Here's how the part is built. I have some questions about the finished solid (model axes, mm). A direction names the side the tool comes from. Coordinates: 2 decimals unless noted, no trailing zeros. Write each loop counter-clockwise with the first axis right and the second up, starting at its lowest first coordinate (ties: lowest second). Pieces come first, ordered by that corner, then holes. Notation, with made-up numbers: (-38, 89.5) -> (-13, 89.5) arc R16 cw to (-13, 115.5) -> close; hole circle Ø6 at (-14.75, 13.5). An arc over 180 degrees is marked (long way). Use a Markdown table: item, result. Add a question column.
Item 1: Will these pins go through, and if not, where does the flat tip stop? pin 1 Ø1.6 at (x, y) = (73.5, 70) entering from +Z; pin 2 Ø3.5 at (x, y) = (14.5, 61.2) entering from +Z.
Item 2: Imagine slicing it at D-D, the plane x = 60.5. Write out the boundary of the cut face in (y, z).
Item 3: Imagine slicing it at A-A, the plane y = -3. Write out the boundary of the cut face in (x, z), and give its area (3 significant figures).
Item 4: If I drill on line 1 along Y through (x, z) = (14.5, 2.6) (3 decimals); line 2 along X through (y, z) = (35.65, 3.3); line 3 along X through (y, z) = (52, 1.85), over which ranges is the centre line in solid material (lowest first)? Write a range as from..to.
Item 5: On a 3-axis mill with a long thin cutter (end or side, diameter ignored), from which of +Z, -Z, +X, -X, +Y, -Y can I reach the whole of each face in a straight line? I mean faces 1 (the flat face through (45, -6, 5.4)), 2 (the cylindrical face through (9.34, 7.52, 2.94)), 3 (the cylindrical face through (85.9, 9.93, 2.74)). Say none if no direction works.
Item 6: Imagine slicing it at C-C, the plane y = 21.65. Write out the boundary of the cut face in (x, z).
Item 7: If we mould it in two halves opening along X, with no side actions, what happens to faces 4 (the flat face through (64, 10.5, 3)), 5 (the flat face through (60, 47, 5.4))? For each: pulls with the +X half, pulls with the -X half, needs draft (parallel to the pull), parting line crosses it, or undercut.
Item 8: Imagine slicing it at B-B, the plane z = 2.4. Count the separate pieces of the cut face and the enclosed holes in it, and give its area (3 significant figures).
```python
from build123d import *

# Parameters (mm, degrees)
SKETCH1_R           = 2.75
SKETCH1_R_2         = 2.25
BOSS_EXTRUDE1_DEPTH = 5.4
FILLET1_R           = 4
SKETCH2_R           = 3.025
CUT_EXTRUDE1_DEPTH  = 6.4
SKETCH3_R           = 2.25
CUT_EXTRUDE2_DEPTH  = 5
CIRPATTERN1_COUNT   = 2
FILLET2_R           = 2
FILLET3_R           = 2
SKETCH5_W           = 99
SKETCH5_H           = 83.2
SKETCH5_W_2         = 93
SKETCH5_H_2         = 77.2
BOSS_EXTRUDE3_DEPTH = 5.4
SKETCH6_W           = 5
SKETCH6_H           = 2
SKETCH6_W_2         = 2
SKETCH6_H_2         = 5
BOSS_EXTRUDE4_DEPTH = 1


with BuildPart() as part:
    # Sketch1 → Boss-Extrude1 (new body)
    with BuildSketch(Plane.XY):
        Polygon((0, 0), (86.5, 0), (86.5, 10.5), (39, 10.5), (39, 50.8), (0, 50.8), align=None)
        with Locations((56.5, 6)):
            Circle(SKETCH1_R, mode=Mode.SUBTRACT)
        with Locations((11, 17.55)):
            Circle(SKETCH1_R_2, mode=Mode.SUBTRACT)
        with Locations((80.5, 6)):
            Circle(SKETCH1_R, mode=Mode.SUBTRACT)
        with Locations((11, 45.55)):
            Circle(SKETCH1_R_2, mode=Mode.SUBTRACT)
        with Locations((35, 31.55)):
            Circle(SKETCH1_R_2, mode=Mode.SUBTRACT)
    extrude(amount=BOSS_EXTRUDE1_DEPTH)

    # Fillet1
    fillet1_edges = [part.edges().sort_by_distance(p)[0] for p in [
        (39, 10.5, 2.7),
    ]]
    fillet(fillet1_edges, radius=FILLET1_R)

    # Sketch2 → Cut-Extrude1 (cut, through all)
    with BuildSketch(Plane.XY.offset(5.4)):
        with Locations((68.5, 6)):
            Circle(SKETCH2_R)
    extrude(amount=-CUT_EXTRUDE1_DEPTH, mode=Mode.SUBTRACT)

    # Sketch3 → Cut-Extrude2 (cut)
    with BuildSketch(Plane.XY.offset(5.4)):
        with Locations((11, 6)):
            Circle(SKETCH3_R)
        with Locations((35, 6)):
            Circle(SKETCH3_R)
    extrude(amount=-CUT_EXTRUDE2_DEPTH, mode=Mode.SUBTRACT)


with BuildPart() as cirpattern1_1:
    # CirPattern1: pattern copy
    add(part.part.rotate(Axis((41.5, 33.6, 0), (0, 0, 1)), 1 * 360 / CIRPATTERN1_COUNT))

    # Fillet2
    fillet2_edges = [cirpattern1_1.edges().sort_by_distance(p)[0] for p in [
        (83, 16.4, 2.7),
        (44, 16.4, 2.7),
        (-3.5, 56.7, 2.7),
        (-3.5, 67.2, 2.7),
        (83, 67.2, 2.7),
    ]]
    fillet(fillet2_edges, radius=FILLET2_R)


with BuildPart() as part_1:
    add(part.part)

    # Fillet3
    fillet3_edges = [part_1.edges().sort_by_distance(p)[0] for p in [
        (0, 50.8, 2.7),
        (39, 50.8, 2.7),
        (86.5, 10.5, 2.7),
        (86.5, 0, 2.7),
        (0, 0, 2.7),
    ]]
    fillet(fillet3_edges, radius=FILLET3_R)

    add(cirpattern1_1.part)  # Boss-Extrude4 merges CirPattern1_1


with BuildPart() as body_3:
    # Sketch5 → Boss-Extrude3 (new body)
    with BuildSketch(Plane(origin=(0, 0, 0), x_dir=(-1, 0, 0), z_dir=(0, 0, -1))):
        with Locations((-41.5, 33.6)):
            Rectangle(SKETCH5_W, SKETCH5_H)
        with Locations((-41.5, 33.6)):
            Rectangle(SKETCH5_W_2, SKETCH5_H_2, mode=Mode.SUBTRACT)
    extrude(amount=-BOSS_EXTRUDE3_DEPTH)


with BuildPart() as part_2:
    add(part_1.part)

    add(body_3.part)  # Boss-Extrude4 merges body 3
    # Sketch6 → Boss-Extrude4 (add)
    with BuildSketch(Plane(origin=(0, 0, 0), x_dir=(-1, 0, 0), z_dir=(0, 0, -1))):
        with Locations((-41.5, 33.6)):
            Rectangle(SKETCH6_W, SKETCH6_H)
        with Locations((2.5, 41.8)):
            Rectangle(SKETCH6_W, SKETCH6_H)
        with Locations((-9, -2.5)):
            Rectangle(SKETCH6_W_2, SKETCH6_H_2)
        with Locations((-77.5, -2.5)):
            Rectangle(SKETCH6_W_2, SKETCH6_H_2)
        with Locations((-85.5, 25.4)):
            Rectangle(SKETCH6_W, SKETCH6_H)
        with Locations((-74, 69.7)):
            Rectangle(SKETCH6_W_2, SKETCH6_H_2)
        with Locations((-5.5, 69.7)):
            Rectangle(SKETCH6_W_2, SKETCH6_H_2)
    extrude(amount=-BOSS_EXTRUDE4_DEPTH)


solid = part_2.part
```
Ans:
| question | item | result |
|---|---|---|
| 1 | pin 1 | stops at z = 1 |
| 1 | pin 2 | passes through |
| 2 | outline | (-8, 0) -> (-5, 0) -> (-5, 5.4) -> (-8, 5.4) -> close; (0, 0) -> (10.5, 0) -> (10.5, 5.4) -> (0, 5.4) -> close; (16.4, 0) -> (67.2, 0) -> (67.2, 5.4) -> (16.4, 5.4) -> close; (72.2, 0) -> (75.2, 0) -> (75.2, 5.4) -> (72.2, 5.4) -> close |
| 3 | outline | (-8, 0) -> (-5, 0) -> (-5, 5.4) -> (-8, 5.4) -> close; (8, 0) -> (10, 0) -> (10, 1) -> (8, 1) -> close; (76.5, 0) -> (78.5, 0) -> (78.5, 1) -> (76.5, 1) -> close; (88, 0) -> (91, 0) -> (91, 5.4) -> (88, 5.4) -> close |
| 3 | area | 36.4 mm^2 |
| 4 | line 1 | y = -8..-5, 0..50.8, 56.7..58.175, 64.225..67.2, 72.2..75.2 |
| 4 | line 2 | x = -8..-5, 0..39, 44..45.75, 50.25..83, 88..91 |
| 4 | line 3 | x = -8..-5, 44..83, 88..91 |
| 5 | face 1 | +Z, +X, -X, +Y, -Y |
| 5 | face 2 | +Z |
| 5 | face 3 | +Z, -Z |
| 6 | outline | (-8, 0) -> (-5, 0) -> (-5, 5.4) -> (-8, 5.4) -> close; (0, 0) -> (39, 0) -> (39, 5.4) -> (0, 5.4) -> close; (44, 0) -> (69.75, 0) -> (69.75, 5.4) -> (44, 5.4) -> close; (74.25, 0) -> (83, 0) -> (83, 5.4) -> (74.25, 5.4) -> close; (88, 0) -> (91, 0) -> (91, 5.4) -> (88, 5.4) -> close |
| 7 | face 4 | undercut |
| 7 | face 5 | needs draft |
| 8 | separate pieces | 3 |
| 8 | enclosed holes | 17 |
| 8 | area | 5,700 mm^2 |
